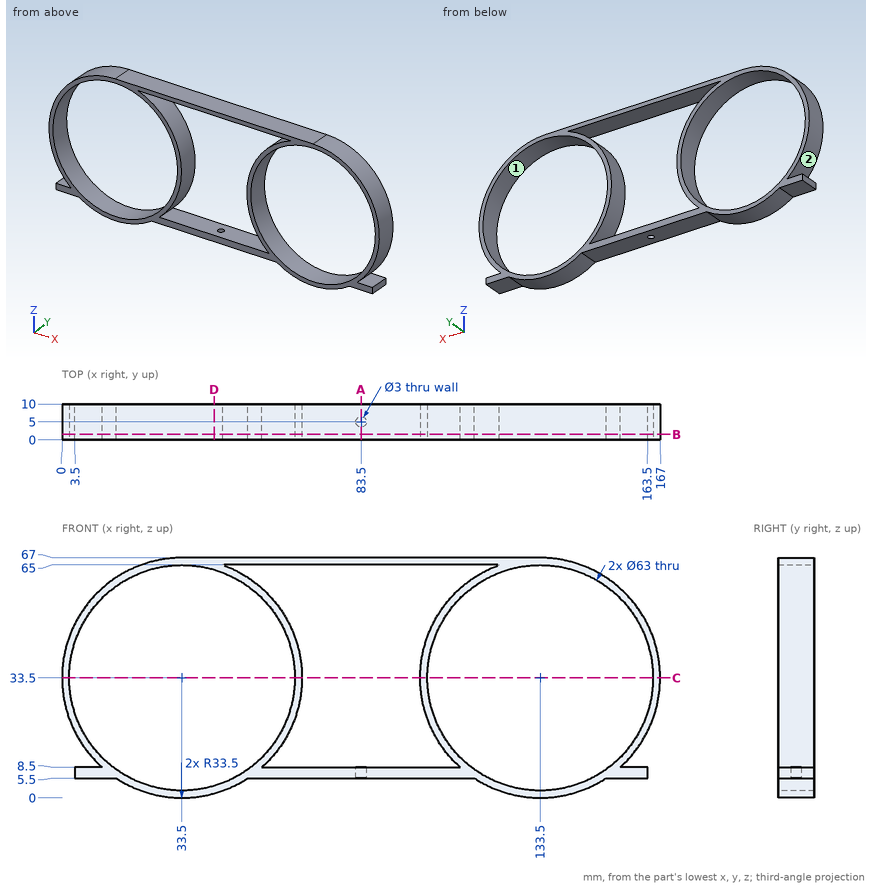
Answer from the drawing. Dimensions are ordinates in mm from the lowest x, y and z of the part. Coordinates: 2 decimals unless noted, no trailing zeros. Write each loop counter-clockwise with the first axis right and the second up, starting at its lowest first coordinate (ties: lowest second). Pieces come first, ordered by that corner, then holes. Notation, with made-up numbers: (67.5, -36.5) - (91.5, -36.5) arc R27 ccw to (91.5, -5.5) - close; hole circle Ø6 at (9, 1). An arc over 180 degrees is marked (long way). Return JSON: item names as keys, results as strings.
1. Consider line 1 along X through (y, z) = (6.5, 33.5); line 2 along X through (y, z) = (7, 45); line 3 along Y through (x, z) = (83.5, 6.2). Determine where each line is inside the solid, lowest interval first.
Final values:
{"line 1": "0 to 2, 65 to 67, 100 to 102, 165 to 167", "line 2": "2.04 to 4.17, 62.83 to 64.96, 102.04 to 104.17, 162.83 to 164.96", "line 3": "0 to 3.5, 6.5 to 10"}
2. The part is cut by section C-C on z = 33.5. Determine the outline of the cut face in (x, y), then the cut area to 3 significant figures.
Final values:
{"outline": "(0, 0) - (2, 0) - (2, 10) - (0, 10) - close; (65, 0) - (67, 0) - (67, 10) - (65, 10) - close; (100, 0) - (102, 0) - (102, 10) - (100, 10) - close; (165, 0) - (167, 0) - (167, 10) - (165, 10) - close", "area": "80.0 mm^2"}
3. Each of these flat-tipped pins is pushed along its axis until it touches: pin 1 Ø3 at (x, y) = (88.5, 4) entering from -Z; pin 2 Ø4 at (x, y) = (8, 7) entering from +Z; pin 3 Ø12 at (x, z) = (121, 53) entering from -Y; pin 4 Ø1 at (y, z) = (8.5, 23) entering from -X. Where does it stop, or does it pass through?
Final values:
{"pin 1": "z = 5.5", "pin 2": "z = 57.37", "pin 3": "through", "pin 4": "x = 1.53"}
4. The part is cut by section B-B on y = 1.5. Determine the outline of the cut face in (x, z), then the cut area to 3 significant figures.
Final values:
{"outline": "(3.5, 5.5) - (15.11, 5.5) arc R33.5 ccw to (51.89, 5.5) - (115.11, 5.5) arc R33.5 ccw to (151.89, 5.5) - (163.5, 5.5) - (163.5, 8.5) - (155.8, 8.5) arc R33.5 ccw to (133.5, 67) - (33.5, 67) arc R33.5 ccw to (11.2, 8.5) - (3.5, 8.5) - close; hole circle Ø63 at (33.5, 33.5); hole (44.9, 65) arc R33.5 cw to (55.8, 8.5) - (111.2, 8.5) arc R33.5 cw to (122.1, 65) - close; hole circle Ø63 at (133.5, 33.5)", "area": "1,220 mm^2"}
5. For a pull along X with two mould halves and no side action, classify the marked faces 1 and 2 as +X half, -X half, draft (parallel to the pull), parting line (faces both ways), or undercut.
Final values:
{"face 1": "undercut", "face 2": "-X half"}
6. The part is cut by section A-A on x = 83.5. Determine the outline of the cut face in (y, z).
Final values:
{"outline": "(0, 5.5) - (3.5, 5.5) - (3.5, 8.5) - (0, 8.5) - close; (0, 65) - (10, 65) - (10, 67) - (0, 67) - close; (6.5, 5.5) - (10, 5.5) - (10, 8.5) - (6.5, 8.5) - close"}
7. The part is cut by section D-D on x = 42.5. Determine the outline of the cut face in (y, z).
Final values:
{"outline": "(0, 1.23) - (10, 1.23) - (10, 3.31) - (0, 3.31) - close; (0, 63.69) - (10, 63.69) - (10, 67) - (0, 67) - close"}
